Model file for the job. Use its own axes, mm. A direction names the side the tool comes from. Coordinates: 2 decimals unless noted, no trailing zeros. Loops run counter-clockwise (first coordinate to the right, second up) from the corner with the lowest first, then second, coordinate; pieces in that order, holes last.
from build123d import *

# Parameters (mm, degrees)
F0_R     = 63.5
F1_DEPTH = 50.8
F2_W     = 50.8
F2_H     = 25.4
F3_DEPTH = 50.8
F5_D     = 6.35
F6_R     = 5.08
F7_R     = 5.08
F8_W     = 12.7
F8_H     = 25.4


# Not quite as in the source:
# - a pattern or mirror of a feature is missing from the dataset's text; its kind, count and spacing are read off the source's solid


with BuildPart() as f1:
    # F0 (on Top) → F1 (new body, symmetric)
    with BuildSketch(Plane.XY):
        Circle(F0_R)
    extrude(amount=F1_DEPTH, both=True)

    # F2 (on face) → F3 (cut)
    with BuildSketch(Plane.XY.offset(50.8)):
        Rectangle(F2_W, F2_H)
    extrude(amount=-F3_DEPTH, mode=Mode.SUBTRACT)

    # F5 (through all)
    with Locations(Plane(origin=(0, 0, -50.8), x_dir=(1, 0, 0), z_dir=(0, 0, -1))):
        with Locations((0, 0)):
            Hole(F5_D / 2)

    # F6
    f6_edges = [f1.edges().sort_by_distance(p)[0] for p in [
        (-63.5, 0, -50.8),
    ]]
    fillet(f6_edges, radius=F6_R)

    # F7
    f7_edges = [f1.edges().sort_by_distance(p)[0] for p in [
        (-25.4, 0, 0),
    ]]
    fillet(f7_edges, radius=F7_R)

    # F8 (on Front) → F9 (revolve)
    with BuildSketch(Plane.XZ):
        with Locations((-31.75, -63.5)):
            Rectangle(F8_W, F8_H)
    f9 = revolve(axis=Axis((0, 0, 19.3926589563), (0, 0, -1)))

    # F9_copies: F9 across plane
    add(f9.mirror(Plane.XY))


solid = f1.part
Q1. Which spindle directions (+Z, -Z, +X, -X, +Y, -Y) get a long thin tool onto all of the face, cutting with end or side? Do faces 4 (the cylindrical face through (0.69, 3.1, -25.04)), 5 (the cylindrical face through (5.506, -24.796, -63.322)), 6 (the cylindrical face through (5.506, -24.796, 63.322)), 7 (the flat face through (25.4, 0, 26)), 8 (the flat face through (-25, -8, -76.2)). Say none if no direction does.
Answers:
face 4: +Z, -Z
face 5: -Z
face 6: +Z
face 7: none
face 8: -Z, +X, -X, +Y, -Y
Q2. Mould opens along X. For faces 1 (the cylindrical face through (-13.77, -61.99, 3.22)), 2 (the cylindrical face through (-23.951, 0.178, 1.528)), 3 (the flat face through (-25, -8, 76.2)) say: +X half, -X half, draft (parallel to the pull), parting line (faces both ways), or undercut.
Answers:
face 1: parting line
face 2: undercut
face 3: draft
Q3. Slice it at B-B (z = 31). List the corners of the cut face in (x, y).
Answers:
outline: circle Ø127 at (0, 0); hole (-25.4, -12.7) - (25.4, -12.7) - (25.4, 12.7) - (-25.4, 12.7) - close
Q4. Drill centre lines: line 1 (Y direction, x = 0, z = -66); line 2 (Y direction, x = 0, z = -10.5) (3 decimals); line 3 (Z direction, x = -13, y = 41). Where is each one in solid material? Low to high.
Answers:
line 1: y = -38.1 to -25.4, 25.4 to 38.1
line 2: y = -63.5 to -3.175, 3.175 to 63.5
line 3: z = -50.8 to 50.8
Q5. Slice it at D-D (z = -33). List the corners of the cut face in (x, y) (3 decimals).
Answers:
outline: circle Ø127 at (0, 0); hole circle Ø6.35 at (0, 0)
Q6. Flat gauge pins, fed straight in: P1, Ø5, axis at x = 51, z = -29.5, coming from the -Y side; P2, Ø1.5, axis at x = -28.5, y = 40.5, coming from the -Z side; P3, Ø3, axis at x = 42, z = 40.5, coming from the -Y side. Where does each tip first touch, or does it go through?
Answers:
P1: stops at y = -40.99
P2: stops at z = -50.8
P3: stops at y = -48.91
Q7. Slice it at C-C (z = -67). List the corners of the cut face in (x, y).
Answers:
outline: circle Ø76.2 at (0, 0); hole circle Ø50.8 at (0, 0)
